from build123d import *

# Parameters (mm, degrees)
SKETCH2_W           = 120
SKETCH2_H           = 120
BOSS_EXTRUDE1_DEPTH = 90
FILLET1_R           = 10
SHELL1_T            = -4
CUT_EXTRUDE1_DEPTH  = 20


with BuildPart() as part:
    # Sketch2 → Boss-Extrude1 (new body)
    with BuildSketch(Plane.XY):
        with Locations((60, 60)):
            Rectangle(SKETCH2_W, SKETCH2_H)
    extrude(amount=BOSS_EXTRUDE1_DEPTH)

    # Fillet1
    fillet1_edges = [part.edges().sort_by_distance(p)[0] for p in [
        (0, 120, 45),
        (120, 120, 45),
        (120, 0, 45),
        (0, 0, 45),
    ]]
    fillet(fillet1_edges, radius=FILLET1_R)

    # Shell1
    shell1_openings = [part.faces().sort_by_distance(p)[0] for p in [
        (60, 60, 90),
    ]]
    offset(amount=SHELL1_T, openings=shell1_openings, kind=Kind.INTERSECTION)

    # Sketch4 → Cut-Extrude1 (cut)
    with BuildSketch(Plane.XY.offset(90)):
        with BuildLine():
            Line((0, 110), (0, 10))
            ThreePointArc((0, 10), (2.928932188, 2.928932188), (10, 0))
            Line((10, 0), (110, 0))
            ThreePointArc((110, 0), (117.071067812, 2.928932188), (120, 10))
            Line((120, 10), (120, 110))
            ThreePointArc((120, 110), (117.071067812, 117.071067812), (110, 120))
            Line((110, 120), (10, 120))
            ThreePointArc((10, 120), (2.928932188, 117.071067812), (0, 110))
        make_face()
        with BuildLine():
            Line((2.2, 110), (2.2, 10))
            ThreePointArc((2.2, 10), (4.484567107, 4.484567107), (10, 2.2))
            Line((10, 2.2), (110, 2.2))
            ThreePointArc((110, 2.2), (115.515432893, 4.484567107), (117.8, 10))
            Line((117.8, 10), (117.8, 110))
            ThreePointArc((117.8, 110), (115.515432893, 115.515432893), (110, 117.8))
            Line((110, 117.8), (10, 117.8))
            ThreePointArc((10, 117.8), (4.484567107, 115.515432893), (2.2, 110))
        make_face(mode=Mode.SUBTRACT)
    extrude(amount=-CUT_EXTRUDE1_DEPTH, mode=Mode.SUBTRACT)


solid = part.part
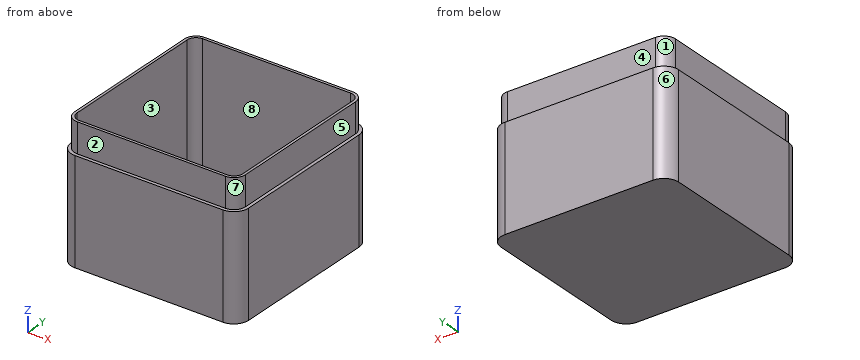
The listing builds one solid part. Answer for the finished solid, in the listing's coordinates (mm). Face numbers are marked on the shaded views. A direction names the side the tool comes from. Give positions to 0.01 mm unless a question says otherwise; leave off trailing zeros. Loops run counter-clockwise (first coordinate to the right, second up) from the corner with the lowest first, then second, coordinate; pieces in that order, holes last. Notation, with made-up numbers: (-34, -15.75) - (-17, -15.75) arc R26 ccw to (-17, 12.25) - close; hole circle Ø9 at (58, 63.25). An arc over 180 degrees is marked (long way). Use one line per item in the form item = value.
1. Section A-A on z = 17 is taken. Give the vertices of the cut face in (x, y).
Calculated:
outline = (0, 10) arc R10 ccw to (10, 0) - (110, 0) arc R10 ccw to (120, 10) - (120, 110) arc R10 ccw to (110, 120) - (10, 120) arc R10 ccw to (0, 110) - close; hole (4, 10) arc R6 ccw to (10, 4) - (110, 4) arc R6 ccw to (116, 10) - (116, 110) arc R6 ccw to (110, 116) - (10, 116) arc R6 ccw to (4, 110) - close
2. Find the intervals of material crossed by line 1 along X through (y, z) = (14.5, 40.5); line 2 along Y through (x, z) = (29, 86), in increasing order. Write a range as [from, to].
Calculated:
line_1 = [0, 4], [116, 120]
line_2 = [2.2, 4], [116, 117.8]
3. Given pin 1 Ø10 at (x, z) = (64.5, 76) entering from -Y; pin 2 Ø1.5 at (x, y) = (101, 81.5) entering from +Z; pin 3 Ø10 at (y, z) = (44.5, 75.5) entering from +X, each flat-ended and moving along its own axis, determine where each tip first touches the part or whether it passes through.
Calculated:
pin_1 = 2.2
pin_2 = 4
pin_3 = 117.8
4. Section D-D on z = 79 is taken. Give the vertices of the cut face in (x, y), then the cut area to 3 significant figures.
Calculated:
outline = (2.2, 10) arc R7.8 ccw to (10, 2.2) - (110, 2.2) arc R7.8 ccw to (117.8, 10) - (117.8, 110) arc R7.8 ccw to (110, 117.8) - (10, 117.8) arc R7.8 ccw to (2.2, 110) - close; hole (4, 10) arc R6 ccw to (10, 4) - (110, 4) arc R6 ccw to (116, 10) - (116, 110) arc R6 ccw to (110, 116) - (10, 116) arc R6 ccw to (4, 110) - close
area = 798 mm^2
5. The mould has two halves that part along Y. Classify the marked faces 6, 7 and 8: pulls with the +Y half, pulls with the -Y half, needs draft (parallel to the pull), parting line crosses it, or undercut.
Calculated:
face_6 = pulls with the +Y half
face_7 = pulls with the -Y half
face_8 = undercut
6. Which of the six approach directions +Z, -Z, +X, -X, +Y, -Y give full straight-line access (tool end or side, diameter ignored) to the marked faces 1, 2, 3, 4 and 5?
Calculated:
face_1 = +Z, -X, +Y
face_2 = +Z, +X, -X, -Y
face_3 = +Z
face_4 = +Z, +X, -X, +Y
face_5 = +Z, +X, +Y, -Y
7. Section B-B on y = 21.5 is taken. Give the vertices of the cut face in (x, z), then the cut area to 3 significant figures.
Calculated:
outline = (0, 0) - (120, 0) - (120, 70) - (117.8, 70) - (117.8, 90) - (116, 90) - (116, 4) - (4, 4) - (4, 90) - (2.2, 90) - (2.2, 70) - (0, 70) - close
area = 1,080 mm^2
